Check sheet for the modelled part. Datum: model origin and axes. Units: mm. Face numbers are marked on the shaded views. Give positions to 0.01 mm unless a question says otherwise; leave off trailing zeros. Loops run counter-clockwise (first coordinate to the right, second up) from the corner with the lowest first, then second, coordinate; pieces in that order, holes last. Notation, with made-up numbers: (62.25, 13.25) - (114.25, 13.25) arc R25 cw to (114.25, 25.25) - close; hole circle Ø4 at (87, -30.75). An arc over 180 degrees is marked (long way). Use CSV: the item, a comma, the result in double quotes.
from build123d import *

# Parameters (mm, degrees)
ESQUISSE1_W      = 145
ESQUISSE1_H      = 79
EXTRUSION1_DEPTH = 5
EXTRUSION2_REACH = 108.696
ESQUISSE2_W      = 60
ESQUISSE2_H      = 10


with BuildPart() as part:
    # Esquisse1 → Extrusion1 (new body)
    with BuildSketch(Plane(origin=(0, 0, 0), x_dir=(1, 0, 0), z_dir=(0, 1, 0))):
        with Locations((24.232219602, -5.242282495)):
            Rectangle(ESQUISSE1_W, ESQUISSE1_H)
    extrude(amount=EXTRUSION1_DEPTH)

    # Esquisse2 → Extrusion2 (cut, up to next)
    with BuildSketch(Plane(origin=(0, 5, 0), x_dir=(1, 0, 0), z_dir=(0, 1, 0)), mode=Mode.PRIVATE) as extrusion2_sk1:
        with Locations((52.732219602, 29.257717505)):
            Rectangle(ESQUISSE2_W, ESQUISSE2_H)
    extrusion2_tool1 = extrude(extrusion2_sk1.sketch, amount=-EXTRUSION2_REACH, mode=Mode.PRIVATE) & part.part
    # Esquisse2 → Extrusion2 (cut, up to next)
    with BuildSketch(Plane(origin=(0, 5, 0), x_dir=(1, 0, 0), z_dir=(0, 1, 0)), mode=Mode.PRIVATE) as extrusion2_sk2:
        with Locations((52.732219602, -39.742282495)):
            Rectangle(ESQUISSE2_W, ESQUISSE2_H)
    extrusion2_tool2 = extrude(extrusion2_sk2.sketch, amount=-EXTRUSION2_REACH, mode=Mode.PRIVATE) & part.part
    add(extrusion2_tool1.solids().sort_by_distance((52.73222, 5, -29.257718))[0], mode=Mode.SUBTRACT)
    add(extrusion2_tool2.solids().sort_by_distance((52.73222, 5, 39.742282))[0], mode=Mode.SUBTRACT)


solid = part.part
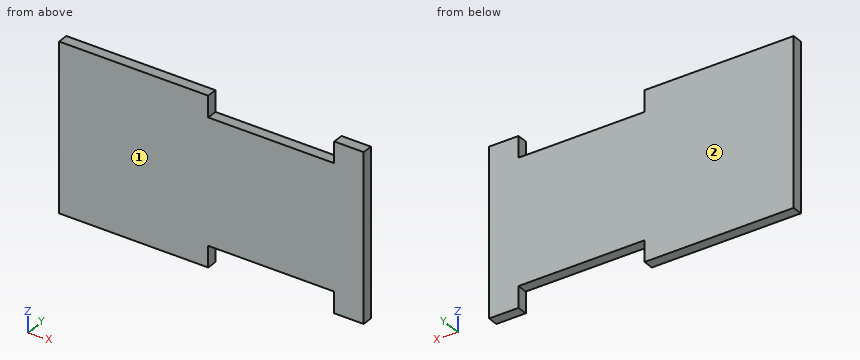
1. Sectioned sample at C-C, the plane x = 33. Record the boundary of the cut face in (y, z), and give its area (3 significant figures).
Completed:
outline,"(0, -24.26) - (5, -24.26) - (5, 34.74) - (0, 34.74) - close"
area,"295 mm²"
2. Sectioned sample at B-B, the plane y = 2.9. Record the boundary of the cut face in (x, z).
Completed:
outline,"(-48.27, -34.26) - (22.73, -34.26) - (22.73, -24.26) - (82.73, -24.26) - (82.73, -34.26) - (96.73, -34.26) - (96.73, 44.74) - (82.73, 44.74) - (82.73, 34.74) - (22.73, 34.74) - (22.73, 44.74) - (-48.27, 44.74) - close"
3. Release check for a two-part mould opening along Y. For the marked faces 1 and 2 record: released by +Y, released by -Y, zero draft, split by the parting line, or undercut.
Completed:
face 1,"released by -Y"
face 2,"released by +Y"
4. Sectioned sample at A-A, the plane z = 39. Record the boundary of the cut face in (x, y), and give its area (3 significant figures).
Completed:
outline,"(-48.27, 0) - (22.73, 0) - (22.73, 5) - (-48.27, 5) - close; (82.73, 0) - (96.73, 0) - (96.73, 5) - (82.73, 5) - close"
area,"425 mm²"
5. Scan lines: line 1 along X through (y, z) = (0.4, 35.5); line 2 along Z through (x, y) = (68, 1.9). Record each from-to range of solid material in increasing order.
Completed:
line 1,"x = -48.27 to 22.73, 82.73 to 96.73"
line 2,"z = -24.26 to 34.74"
